For this review, take the finished solid that the model builds, in its own axes (mm). Face numbers are marked on the shaded views. A direction names the side the tool comes from. Give positions to 0.01 mm unless a question says otherwise; leave off trailing zeros. Loops run counter-clockwise (first coordinate to the right, second up) from the corner with the lowest first, then second, coordinate; pieces in that order, holes last. Notation, with made-up numbers: (22.25, -35) -> (30.25, -35) arc R13 cw to (30.25, -18) -> close; hole circle Ø9 at (29, 43.5). An arc over 180 degrees is marked (long way). Answer as CSV lines item,"result". Start each with the question number.
Item 1: Machinability: for the marked faces 4 and 5, which of the approach directions +Z, -Z, +X, -X, +Y, -Y give a long, thin tool a straight path to every point of the face, cutting with its end or side? Answer none if there is none.
Item 2: Add section B-B on z = 0. State the section outline as (x, y) points (3 decimals), plus the area to 3 significant figures.
Item 3: For L1, parallel to X at y = -9, z = -20; L2, parallel to Z at x = 0, y = -12; L3, parallel to Z at x = 0, y = 7.5, list the stretches that pass through material, from the lowest coordinate up. Write a range as from..to.
Item 4: Add section A-A on x = 20. State the section outline as (y, z) points.
Item 5: Clearance check with flat-ended pins moving along their axes: P1, Ø7, axis at x = 0, z = 0, coming from the +Y side; P2, Ø7, axis at x = -20, z = -20, coming from the -Y side; P3, Ø10, axis at x = 20, z = -20, coming from the -Y side; P4, Ø15, axis at x = -6, z = 2, coming from the +Y side. State where each tip first meets the part, or that it passes through.
Item 6: The part is to be moulded in two halves that separate along Z. For the marked faces 1, 2 and 3, say which applies: +Z half, -Z half, draft (parallel to the pull), parting line (faces both ways), or undercut.
Item 7: Add section C-C on y = 10. State the section outline as (x, z) points, plus the area to 3 significant figures.
Item 8: Add section D-D on z = -20. State the section outline as (x, y) points.
Solid Edge part; units mm, degrees
sketch "Sketch1" plane through (0, 0, 0) normal (0, -1, 0) x (1, 0, 0)
  line L0 (-32.5, 32.5) -> (32.5, 32.5)
  line L1 (32.5, 32.5) -> (32.5, -32.5)
  line L2 (32.5, -32.5) -> (-32.5, -32.5)
  line L3 (-32.5, -32.5) -> (-32.5, 32.5)
  dimension "D1" = 32.5
  dimension "D2" = 32.5
extrude "Protrusion1" add sketch "Sketch1" along normal mid plane 40
hole "Bohrung_1" at (-20, -20, -20) direction (0, 1, 0) diameter 8.5 depth 50
hole "Hole1" at (20, -20, -20) direction (0, 1, 0) diameter 8.5 depth 50
hole "Hole2" at (0, -20, 20) direction (0, 1, 0) diameter 8.5 depth 50
hole "Bohrung_4" at (0, 20, 0) direction (0, -1, 0) diameter 16 depth 20
hole "Bohrung_5" at (0, -20, 0) direction (0, 1, 0) diameter 5.5 depth 20 countersink diameter 9.73 countersink angle 82
chamfer "Fase_1" distance 1 angle 45 6 edges at (0, -20, 24.25) (0, 20, 15.75) (-20, -20, -15.75) (-20, 20, -24.25) (20, -20, -15.75) (20, 20, -24.25)
chamfer "Fase_3" distance 1 angle 45 12 edges at (0, -20, -32.5) (32.5, -20, 0) (32.5, 0, -32.5) (32.5, 0, 32.5) (-32.5, 0, 32.5) (0, -20, 32.5) (-32.5, -20, 0) (-32.5, 0, -32.5) (-32.5, 20, 0) (0, 20, -32.5) (32.5, 20, 0) (0, 20, 32.5)
hole "Bohrung_6" at (0, 20, 0) direction (0, -1, 0) diameter 30 depth 6
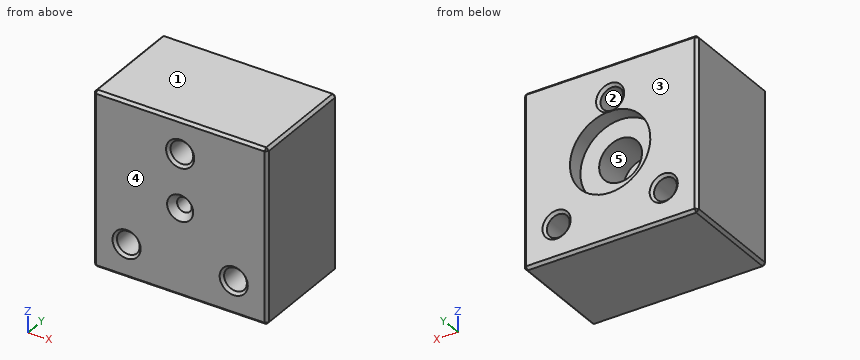
Computed values:
1,face 4,"+Z, -Z, +X, -X, -Y"
1,face 5,"+Y"
2,outline,"(-32.5, -19) -> (-31.5, -20) -> (-4.865, -20) -> (-2.75, -17.567) -> (-2.75, 0) -> (-8, 0) -> (-8, 14) -> (-15, 14) -> (-15, 20) -> (-31.5, 20) -> (-32.5, 19) -> close; (2.75, -17.567) -> (4.865, -20) -> (31.5, -20) -> (32.5, -19) -> (32.5, 19) -> (31.5, 20) -> (15, 20) -> (15, 14) -> (8, 14) -> (8, 0) -> (2.75, 0) -> close"
2,area,"2,080 mm²"
3,L1,"-32.5..-24.25, -15.75..15.75, 24.25..32.5"
3,L2,"-32.5..-2.75, 2.75..15.75, 24.25..32.5"
3,L3,"-32.5..-8, 8..15.75, 24.25..32.5"
4,outline,"(-20, -31.5) -> (-19, -32.5) -> (19, -32.5) -> (20, -31.5) -> (20, -25.25) -> (19, -24.25) -> (-19, -24.25) -> (-20, -25.25) -> close; (-20, -14.75) -> (-19, -15.75) -> (19, -15.75) -> (20, -14.75) -> (20, 31.5) -> (19, 32.5) -> (-19, 32.5) -> (-20, 31.5) -> close"
5,P1,"y = 0"
5,P2,"through"
5,P3,"y = -19.75"
5,P4,"y = 14"
6,face 1,"+Z half"
6,face 2,"undercut"
6,face 3,"draft"
7,outline,"(-32.5, -31.5) -> (-31.5, -32.5) -> (31.5, -32.5) -> (32.5, -31.5) -> (32.5, 31.5) -> (31.5, 32.5) -> (-31.5, 32.5) -> (-32.5, 31.5) -> close; hole circle Ø8.5 at (-20, -20); hole circle Ø16 at (0, 0); hole circle Ø8.5 at (0, 20); hole circle Ø8.5 at (20, -20)"
7,area,"3,850 mm²"
8,outline,"(-32.5, -19) -> (-31.5, -20) -> (-25.25, -20) -> (-24.25, -19) -> (-24.25, 19) -> (-25.25, 20) -> (-31.5, 20) -> (-32.5, 19) -> close; (-15.75, -19) -> (-14.75, -20) -> (14.75, -20) -> (15.75, -19) -> (15.75, 19) -> (14.75, 20) -> (-14.75, 20) -> (-15.75, 19) -> close; (24.25, -19) -> (25.25, -20) -> (31.5, -20) -> (32.5, -19) -> (32.5, 19) -> (31.5, 20) -> (25.25, 20) -> (24.25, 19) -> close"
